Design review of the part built by this model. Coordinates are the model's own, in mm. Coordinates: 2 decimals unless noted, no trailing zeros. Loops run counter-clockwise (first coordinate to the right, second up) from the corner with the lowest first, then second, coordinate; pieces in that order, holes last. Notation, with made-up numbers: M -16,-9.75 L 40,-9.75 A16 cw 40,-2.75 Z; hole C 66.5,88 d2. An arc over 180 degrees is marked long. Answer as CSV lines item,"result". Start each with the question number.
Autodesk Inventor part; units mm, degrees
ref_plane "YZ Plane" through (0, 0, 0) normal (1, 0, 0) x (0, 1, 0)
ref_plane "XZ Plane" through (0, 0, 0) normal (0, 1, 0) x (-1, 0, 0)
ref_plane "XY Plane" through (0, 0, 0) normal (0, 0, 1) x (1, 0, 0)
sketch "Эскиз1" plane through (0, 0, 0) normal (0, 0, 1) x (1, 0, 0)
  line L0 (0, 0) -> (0, 18)
  line L1 (0, 18) -> (100, 18)
  line L2 (100, 18) -> (100, -5)
  line L3 (100, -5) -> (69, -5)
  line L4 (69, -5) -> (69, -12)
  line L5 (69, -12) -> (49, -12)
  line L6 (49, -12) -> (49, 1)
  line L7 (49, 1) -> (32, 1)
  line L8 (32, 1) -> (32, 18)
  line L9 (32, 1) -> (32, -12)
  line L10 (32, -12) -> (49, -12)
  dimension "d7" = 18
  dimension "d8" = 100
  dimension "d9" = 23
  dimension "d10" = 31
  dimension "d11" = 20
  dimension "d12" = 13
  dimension "d13" = 17
  dimension "d26" = 17
revolve "Вращение1" add sketch "Эскиз1" angle 360 about axis through (0, 0, 0) along (0, 1, 0)
sketch "Эскиз2" plane through (0, 18, 0) normal (0, 1, 0) x (1, 0, 0)
  circle A0 centre (0, 0) radius 100
  circle A1 centre (0, 0) radius 100
  line L0 (0, 100) -> (0, 87.5)
  dimension "d15" = 12.5
hole "Отверстие1" at (0, 18, -87.5) direction (0, -1, 0) diameter 12 end through all
pattern_circular "Круговой массив2" count 10 over 360 about axis through (0, 6.5, 0) along (0, -1, 0) of "Отверстие1"
properties part number "Крышка сальников_CPY" material "Чугун, серый"
Item 1: Mouldability with a two-part tool opening along Z and no side actions: class faces 1 (the face through (65.814, -8.549, 20.726)), 2 (the face through (-0.264, 6.339, -93.494)), 3 (the face through (-6.94, 3.21, 31.24)), 4 (the face through (-24, -5, 65)) as released by +Z, released by -Z, zero draft, split by the parting line, or undercut.
Item 2: Add section D-D (y = -8). Give the boundary of the cut face in (x, z), plus the area to 3 significant figures.
Item 3: For pin 1 (8 mm diameter, centred on y = -2.5, z = -48.5, fed in from +X); pin 2 (19 mm diameter, centred on x = -83.22, z = 27.04, fed in from -Y); pin 3 (10 mm diameter, centred on y = 3, z = 46, fed in from +X); pin 4 (7 mm diameter, centred on x = 0, z = 87.5, fed in from -Y), all flat-tipped, find the tip position at first contact; note any pin that passes through.
Item 4: For line 1 along X through (y, z) = (0.5, -22); line 2 along Z through (x, y) = (52, 1.75); line 3 along Y through (x, z) = (68, -39.5), list the stretches that pass through material, from the lowest coordinate up. Write a range as from..to.
Item 5: Add section B-B (x = 0). Give the boundary of the cut face in (y, z), plus the area to 3 significant figures.
Item 6: Add section A-A (z = 0). Give the boundary of the cut face in (x, y), plus the area to 3 significant figures.
Response:
1,face 1,"split by the parting line"
1,face 2,"undercut"
1,face 3,"undercut"
1,face 4,"zero draft"
2,outline,"C 0,0 d138; hole C 0,0 d64"
2,area,"11,700 mm²"
3,pin 1,"x = 89.55"
3,pin 2,"y = -5"
3,pin 3,"x = 91.21"
3,pin 4,"through"
4,line 1,"-97.55..-86.47, -79.96..-23.24, 23.24..79.96, 86.47..97.55"
4,line 2,"-85.42..-76.76, -64.82..64.82, 76.76..85.42"
4,line 3,"-5..18"
5,outline,"M -12,-69 L -5,-69 L -5,-81.5 L 18,-81.5 L 18,-32 L -12,-32 Z; M -12,32 L 18,32 L 18,81.5 L -5,81.5 L -5,69 L -12,69 Z; M -5,-100 L 18,-100 L 18,-93.5 L -5,-93.5 Z; M -5,93.5 L 18,93.5 L 18,100 L -5,100 Z"
5,area,"3,090 mm²"
6,outline,"M -100,-5 L -69,-5 L -69,-12 L -32,-12 L -32,18 L -100,18 Z; M 32,-12 L 69,-12 L 69,-5 L 100,-5 L 100,18 L 32,18 Z"
6,area,"3,650 mm²"
